from build123d import *

# Parameters (mm, degrees)
MODEL_R                 = 16.5
MODEL_R_2               = 3.5
MODEL_R_3               = 2
SALIENTE_EXTRUIR1_DEPTH = 3


with BuildPart() as part:
    # Model → Saliente-Extruir1 (new body)
    with BuildSketch(Plane.XY):
        with Locations((215.747807914, 241.952019993)):
            Circle(MODEL_R)
        with Locations((215.747807914, 232.952019993)):
            Circle(MODEL_R_2, mode=Mode.SUBTRACT)
        with Locations((215.747807914, 250.952019993)):
            Circle(MODEL_R_2, mode=Mode.SUBTRACT)
        with Locations((215.747807914, 241.952019993)):
            Circle(MODEL_R_3, mode=Mode.SUBTRACT)
        with BuildLine():
            ThreePointArc((220.622807913, 239.452019993), (220.842477828, 238.921689907), (221.372807913, 238.702019993))
            Line((221.372807913, 238.702019993), (223.122807913, 238.702019993))
            ThreePointArc((223.122807913, 238.702019993), (223.653137999, 238.921689907), (223.872807913, 239.452019993))
            Line((223.872807913, 239.452019993), (223.872807913, 244.452019993))
            ThreePointArc((223.872807913, 244.452019993), (223.653137999, 244.982350079), (223.122807913, 245.202019993))
            Line((223.122807913, 245.202019993), (221.372807913, 245.202019993))
            ThreePointArc((221.372807913, 245.202019993), (220.842477828, 244.982350079), (220.622807913, 244.452019993))
            Line((220.622807913, 244.452019993), (220.622807913, 239.452019993))
        make_face(mode=Mode.SUBTRACT)
        with BuildLine():
            ThreePointArc((210.122807913, 238.702019993), (210.653137999, 238.921689907), (210.872807913, 239.452019993))
            Line((210.872807913, 239.452019993), (210.872807913, 244.452019993))
            ThreePointArc((210.872807913, 244.452019993), (210.653137999, 244.982350079), (210.122807913, 245.202019993))
            Line((210.122807913, 245.202019993), (208.372807913, 245.202019993))
            ThreePointArc((208.372807913, 245.202019993), (207.842477828, 244.982350079), (207.622807913, 244.452019993))
            Line((207.622807913, 244.452019993), (207.622807913, 239.452019993))
            ThreePointArc((207.622807913, 239.452019993), (207.842477828, 238.921689907), (208.372807913, 238.702019993))
            Line((208.372807913, 238.702019993), (210.122807913, 238.702019993))
        make_face(mode=Mode.SUBTRACT)
    extrude(amount=SALIENTE_EXTRUIR1_DEPTH)


solid = part.part
Design review of the part built by this model. Coordinates are the model's own, in mm. A direction names the side the tool comes from. Give positions to 0.01 mm unless a question says otherwise; leave off trailing zeros. Write each loop counter-clockwise with the first axis right and the second up, starting at its lowest first coordinate (ties: lowest second). Pieces come first, ordered by that corner, then holes. Notation, with made-up numbers: M 24.5,-6.75 L 81.5,-6.75 A29 ccw 81.5,25.25 Z; hole C 2.25,13.25 d4. An arc over 180 degrees is marked long. Answer as a JSON object with one key per item and string values. Group by question number.
1) Tool access review of faces 1 (the face through (216, 239, 3)), 2 (the face through (209, 245.202, 1)): name each direction out of +Z, -Z, +X, -X, +Y, -Y from which nothing blocks a thin tool from reaching the whole face with its end or side.
2) For line 1 along X through (y, z) = (244, 0.2); line 2 along X through (y, z) = (240.5, 0.85); line 3 along Y through (x, z) = (214, 2.1), list the stretches that pass through material, from the lowest coordinate up.
3) We need section D-D (x = 204). Give the boundary of the cut face in (y, z), and give its area (3 significant figures).
4) We need section B-B (x = 222.5). Give the boundary of the cut face in (y, z), and give its area (3 significant figures).
5) Mouldability with a two-part tool opening along X and no side actions: class faces 3 (the face through (216, 239, 0)), 4 (the face through (220.623, 242, 1)), 5 (the face through (213.6, 258.31, 1.48)) as released by +X, released by -X, zero draft, split by the parting line, or undercut.
6) We need section A-A (y = 248.5). Give the boundary of the cut face in (x, z), and give its area (3 significant figures).
7) Clearance check with flat-ended pins moving along their axes: pin 1 Ø1.5 at (y, z) = (248.5, 2) entering from +X; pin 2 Ø1 at (y, z) = (247, 0.5) entering from +X; pin 3 Ø0.9 at (x, z) = (209, 1.5) entering from -Y. State where each tip first meets the part, or that it passes through.
8) We need section C-C (z = 1.5). Give the boundary of the cut face in (x, y).
Answer key:
{
 "1": {"face 1": "+Z, +X, -X, +Y, -Y", "face 2": "+Z, -Z"},
 "2": {"line 1": "x = 199.38 to 207.62, 210.87 to 220.62, 223.87 to 232.12", "line 2": "x = 199.31 to 207.62, 210.87 to 214.37, 217.12 to 220.62, 223.87 to 232.18", "line 3": "y = 225.54 to 229.92, 235.98 to 240.98, 242.92 to 247.92, 253.98 to 258.36"},
 "3": {"outline": "M 230.37,0 L 253.54,0 L 253.54,3 L 230.37,3 Z", "area": "69.5 mm²"},
 "4": {"outline": "M 226.9,0 L 238.7,0 L 238.7,3 L 226.9,3 Z; M 245.2,0 L 257.01,0 L 257.01,3 L 245.2,3 Z", "area": "70.8 mm²"},
 "5": {"face 3": "zero draft", "face 4": "undercut", "face 5": "split by the parting line"},
 "6": {"outline": "M 200.6,0 L 213.25,0 L 213.25,3 L 200.6,3 Z; M 218.25,0 L 230.89,0 L 230.89,3 L 218.25,3 Z", "area": "75.9 mm²"},
 "7": {"pin 1": "stops at x = 231.2", "pin 2": "stops at x = 231.61", "pin 3": "stops at y = 226.7"},
 "8": {"outline": "C 215.75,241.95 d33; hole M 207.62,239.45 A0.75 ccw 208.37,238.7 L 210.12,238.7 A0.75 ccw 210.87,239.45 L 210.87,244.45 A0.75 ccw 210.12,245.2 L 208.37,245.2 A0.75 ccw 207.62,244.45 Z; hole C 215.75,232.95 d7; hole C 215.75,250.95 d7; hole C 215.75,241.95 d4; hole M 220.62,239.45 A0.75 ccw 221.37,238.7 L 223.12,238.7 A0.75 ccw 223.87,239.45 L 223.87,244.45 A0.75 ccw 223.12,245.2 L 221.37,245.2 A0.75 ccw 220.62,244.45 Z"}
}
